```python
from build123d import *

# Parameters (mm, degrees)
F2_R            = 10.5683460292
F3_DEPTH        = 16
F5_DEPTH        = 16
F5_COPIES_COUNT = 14
F8_R            = 13.0683460292
F8_R_2          = 10.5683460292
F9_DEPTH        = 1.5
F10_DEPTH       = 17.501


# Not quite as in the source:
# - a feature of the source that left no trace in its solid (it failed there, or was rolled back) is left out
# - a pattern or mirror of a feature is missing from the dataset's text; its kind, count and spacing are read off the source's solid


with BuildPart() as f3:
    # F2 (on Top) → F3 (new body)
    with BuildSketch(Plane.XY):
        Circle(F2_R)
    extrude(amount=F3_DEPTH)

    # F4 (on face) → F5 (cut, through all)
    with BuildSketch(Plane.XY.offset(16)):
        with BuildLine():
            ThreePointArc((-2.035036184, 10.3705624496), (-1.6695907294, 10.2822178496), (-1.4987572129, 9.9472983692))
            ThreePointArc((-1.4987572129, 9.9472983692), (0, 8.5083460292), (1.4987572129, 9.9472983692))
            ThreePointArc((1.4987572129, 9.9472983692), (1.6695907294, 10.2822178496), (2.035036184, 10.3705624496))
            ThreePointArc((2.035036184, 10.3705624496), (0, 10.5683460292), (-2.035036184, 10.3705624496))
        make_face()
    f5 = extrude(amount=-F5_DEPTH, mode=Mode.SUBTRACT)

    # F5_copies: F5 ×14 about axis
    f5_copies_axis = Axis((0, 0, 0), (0, 0, 1))
    for i in range(1, F5_COPIES_COUNT):
        add(f5.rotate(f5_copies_axis, i * 360 / F5_COPIES_COUNT), mode=Mode.SUBTRACT)

    # F8 (on face) + F2 (on Top) → F9 (join)
    with BuildSketch(Plane.XY):
        Circle(F8_R)
        Circle(F8_R_2, mode=Mode.SUBTRACT)
    with BuildSketch(Plane.XY):
        Circle(F2_R)
    extrude(amount=-F9_DEPTH)

    # F7 (on face) → F10 (cut, through all)
    with BuildSketch(Plane.XY.offset(16)):
        Polygon((3.8393792901, 6.65), (-3.8393792901, 6.65), (-7.6787585802, 0), (-3.8393792901, -6.65), (3.8393792901, -6.65), (7.6787585802, 0), align=None)
    extrude(amount=-F10_DEPTH, mode=Mode.SUBTRACT)


solid = f3.part
```
The model under review builds one solid part; all positions refer to its coordinate system, in mm. A direction names the side the tool comes from. Round coordinates to 2 decimals unless told otherwise and drop trailing zeros. Loops run counter-clockwise (first coordinate to the right, second up) from the corner with the lowest first, then second, coordinate; pieces in that order, holes last. Notation, with made-up numbers: (-5, 80.5) -> (12, 80.5) arc R16 cw to (12, 84.5) -> close; hole circle Ø9 at (-4, 49.25). An arc over 180 degrees is marked (long way). Answer as a JSON object with one key per item and string values. Group by question number.
1) We need section B-B on y = 2.5. Write out the cut boundary in (x, z), then the cut area to 3 significant figures.
2) For line 1 (Y direction, x = -8.75, z = 12.75); line 2 (Y direction, x = -6.5, z = 15.25); line 3 (Z direction, x = -10.75, y = -7.25), list the stretches that pass through material, from the lowest coordinate up. Write a range as [from, to].
3) We need section A-A on x = 0. Write out the cut boundary in (y, z).
4) Mouldability with a two-part tool opening along X and no side actions: class faces 1 (the face through (12.465, 3.925, -0.74)), 2 (the face through (3.66, 7.68, 8.11)), 3 (the face through (6, -6, -1.5)), 4 (the face through (0.03, -8.51, 8.11)) as released by +X, released by -X, zero draft, split by the parting line, or undercut.
5) For faces 5 (the face through (3.721, -7.652, 8.112)), 6 (the face through (-0.03, 8.51, 8.11)), 7 (the face through (0, 6.65, 7)), list the 3-axis set-ups (+Z, -Z, +X, -X, +Y, -Y) from which the entire face can be reached by the end or side of a thin tool; tool diameter is ignored.
6) For pin 1 Ø2 at (x, z) = (4.5, 7) entering from -Y; pin 2 Ø2 at (y, z) = (-5.5, 9) entering from -X; pin 3 Ø3 at (x, y) = (3, 4) entering from -Z; pin 4 Ø4 at (x, z) = (1.5, 5) entering from +Y, all flat-tipped, find the tip position at first contact; note any pin that passes through.
7) We need section C-C on y = 11. Write out the cut boundary in (x, z), then the cut area to 3 significant figures.
Result set:
{
 "1": {"outline": "(-12.83, -1.5) -> (-6.24, -1.5) -> (-6.24, 16) -> (-8.28, 16) -> (-8.28, 0) -> (-12.83, 0) -> close; (6.24, -1.5) -> (12.83, -1.5) -> (12.83, 0) -> (8.28, 0) -> (8.28, 16) -> (6.24, 16) -> close", "area": "85.3 mm²"},
 "2": {"line 1": "[-5.06, -3.34], [-1.12, 1.12], [3.34, 5.06]", "line 2": "[-8.33, -6.94], [-5.54, -2.04], [2.04, 5.54], [6.94, 8.33]", "line 3": "[-1.5, 0]"},
 "3": {"outline": "(-13.07, -1.5) -> (-6.65, -1.5) -> (-6.65, 16) -> (-8.51, 16) -> (-8.51, 0) -> (-13.07, 0) -> close; (6.65, -1.5) -> (13.07, -1.5) -> (13.07, 0) -> (8.51, 0) -> (8.51, 16) -> (6.65, 16) -> close"},
 "4": {"face 1": "split by the parting line", "face 2": "undercut", "face 3": "zero draft", "face 4": "undercut"},
 "5": {"face 5": "+Z", "face 6": "+Z, +Y", "face 7": "+Z, -Z"},
 "6": {"pin 1": "y = -8.06", "pin 2": "x = -9.56", "pin 3": "through", "pin 4": "y = 10.38"},
 "7": {"outline": "(-7.06, -1.5) -> (7.06, -1.5) -> (7.06, 0) -> (-7.06, 0) -> close", "area": "21.2 mm²"}
}
